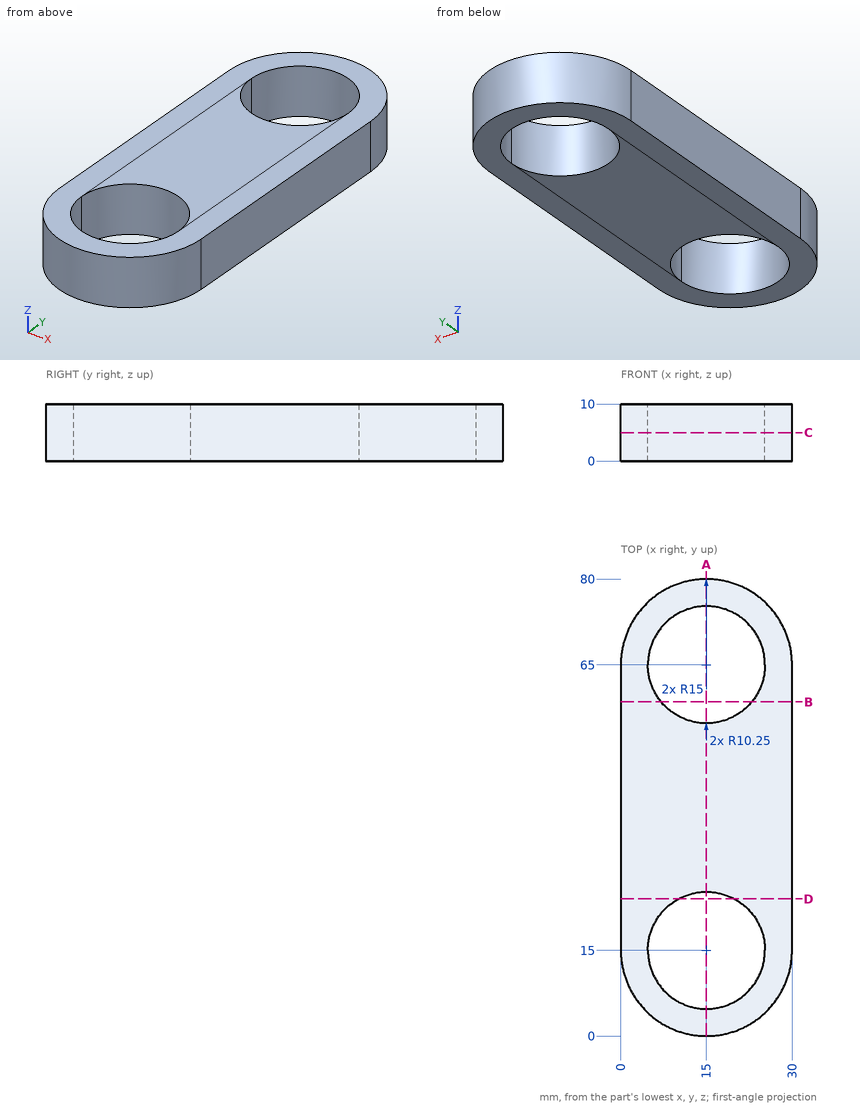
The figure shows three views and two pictorial views of one solid part (mm, origin at its lowest corner). Answer the questions. Give positions to 0.01 mm unless a question says otherwise; leave off trailing zeros. Write each loop counter-clockwise with the first axis right and the second up, starting at its lowest first coordinate (ties: lowest second). Pieces come first, ordered by that corner, then holes. Notation, with made-up numbers: M 58.25,-5.5 L 71.25,-5.5 A31 ccw 71.25,20.5 Z; hole C 34.5,54.5 d3. An arc over 180 degrees is marked long. Write each question's results on one line, items separated by ' | '.
Q1. Section C-C, the plane z = 5 is taken. Write down the section's boundary in (x, y), then the cut area to 3 significant figures.
Output values:
outline: M 0,15 A15 ccw 30,15 L 30,65 A15 ccw 0,65 Z; hole C 15,15 d20.5; hole C 15,65 d20.5 | area: 1,550 mm2
Q2. Section A-A, the plane x = 15 is taken. Write down the section's boundary in (y, z).
Output values:
outline: M 0,0 L 4.75,0 L 4.75,10 L 0,10 Z; M 25.25,0 L 54.75,0 L 54.75,10 L 25.25,10 Z; M 75.25,0 L 80,0 L 80,10 L 75.25,10 Z
Q3. Consider L1, parallel to Y at x = 12.5, z = 9; L2, parallel to Y at x = 14, z = 0.5; L3, parallel to X at y = 19, z = 5.5. Determine where each line is inside the solid, lowest interval first. Write a range as from..to.
Output values:
L1: 0.21..5.06, 24.94..55.06, 74.94..79.79 | L2: 0.03..4.8, 25.2..54.8, 75.2..79.97 | L3: 0..5.56, 24.44..30
Q4. Section D-D, the plane y = 24 is taken. Write down the section's boundary in (x, z).
Output values:
outline: M 0,0 L 10.09,0 L 10.09,10 L 0,10 Z; M 19.91,0 L 30,0 L 30,10 L 19.91,10 Z
Q5. Section B-B, the plane y = 58.5 is taken. Write down the section's boundary in (x, z).
Output values:
outline: M 0,0 L 7.07,0 L 7.07,10 L 0,10 Z; M 22.93,0 L 30,0 L 30,10 L 22.93,10 Z
Q6. Flat-ended cylindrical pins translate along their axes: P1, Ø2, axis at x = 6, z = 7, coming from the +Y side; P2, Ø4, axis at x = 3.5, z = 1, coming from the +Y side. Find the tip coordinate at first contact, or state that the pin passes through.
Output values:
P1: y = 77.69 | P2: y = 76.61
